```python
from build123d import *

# Parameters (mm, degrees)
CHAMFER2_SIZE      = 0.5
CUT_EXTRUDE1_DEPTH = 2


with BuildPart() as part:
    # Sketch1 → Revolve1 (revolve)
    with BuildSketch(Plane.XY):
        Polygon((0, 3), (55, 3), (55, 1.5), (57, 1.5), (57, 2), (62, 2), (62, 0), (-4, 0), (-4, 4.5), (0, 4.5), align=None)
    revolve(axis=Axis((-15.448246648, 0, 0), (1, 0, 0)))

    # Chamfer2
    chamfer2_edges = [part.edges().sort_by_distance(p)[0] for p in [
        (-4, -4.5, 0),
    ]]
    chamfer(chamfer2_edges, length=CHAMFER2_SIZE)

    # Sketch2 → Cut-Extrude1 (cut)
    with BuildSketch(Plane.ZY.offset(4)):
        Polygon((0, 1.732050808), (-1.5, 0.866025404), (-1.5, -0.866025404), (0, -1.732050808), (1.5, -0.866025404), (1.5, 0.866025404), align=None)
    extrude(amount=-CUT_EXTRUDE1_DEPTH, mode=Mode.SUBTRACT)


solid = part.part
```
Build history of the part. All positions in model axes, mm. A direction names the side the tool comes from. Round coordinates to 2 decimals unless told otherwise and drop trailing zeros. Write each loop counter-clockwise with the first axis right and the second up, starting at its lowest first coordinate (ties: lowest second). Pieces come first, ordered by that corner, then holes. Notation, with made-up numbers: (12.25, 23) - (16.25, 23) arc R27 ccw to (16.25, 59) - close; hole circle Ø1 at (68.25, -18.5). An arc over 180 degrees is marked (long way). Write each question's results on one line, items separated by ' | '. Start each with the question number.
Item 1: Mould opens along Z. For faces 1 (the face through (0, 1, -3)), 2 (the face through (-3.014, 1.293, 0.76)), 3 (the face through (60, 0, -2)) say: pulls with the +Z half, pulls with the -Z half, needs draft (parallel to the pull), parting line crosses it, or undercut.
Item 2: Wall check: L1, parallel to X at y = 0.75, z = -3.25; L2, parallel to X at y = -2.75, z = 1; L3, parallel to Z at x = 26.5, y = 0.25. Give the ranges that are in metal, low to high. Write a range as [from, to].
Item 3: Saw through at B-B (x = 16.5). Write the cut outline in (y, z).
Item 4: Saw through at A-A (y = 0). Write the cut outline in (x, z).
Item 5: Which spindle directions (+Z, -Z, +X, -X, +Y, -Y) get a long thin tool onto all of the face, cutting with end or side? Do faces 4 (the face through (-1.73, -0.59, 4.46)), 5 (the face through (56.01, -1.5, 0.07)), 6 (the face through (62, 0, 0)), 7 (the face through (28, -3, 0)), 8 (the face through (-2, 0, 0)). Say none if no direction does.
Item 6: Drop flat-ended pins along their axis: P1, Ø2, axis at x = 44.5, y = -2, coming from the -Z side; P2, Ø2, axis at x = 6.5, y = -3, coming from the +Z side; P3, Ø3, axis at x = 47, z = 0.5, coming from the +Y side. Give the stop position or say it passes through.
Results are:
1) face 1: needs draft | face 2: undercut | face 3: parting line crosses it
2) L1: x = [-4, 0] | L2: x = [-4, 55] | L3: z = [-2.99, 2.99]
3) outline: circle Ø6 at (0, 0)
4) outline: (-4, -4) - (-3.5, -4.5) - (0, -4.5) - (0, -3) - (55, -3) - (55, -1.5) - (57, -1.5) - (57, -2) - (62, -2) - (62, 2) - (57, 2) - (57, 1.5) - (55, 1.5) - (55, 3) - (0, 3) - (0, 4.5) - (-3.5, 4.5) - (-4, 4) - (-4, 1.5) - (-2, 1.5) - (-2, -1.5) - (-4, -1.5) - close
5) face 4: +X, -X | face 5: none | face 6: +Z, -Z, +X, +Y, -Y | face 7: +X | face 8: -X
6) P1: stops at z = -2.83 | P2: stops at z = 2.24 | P3: stops at y = 3
